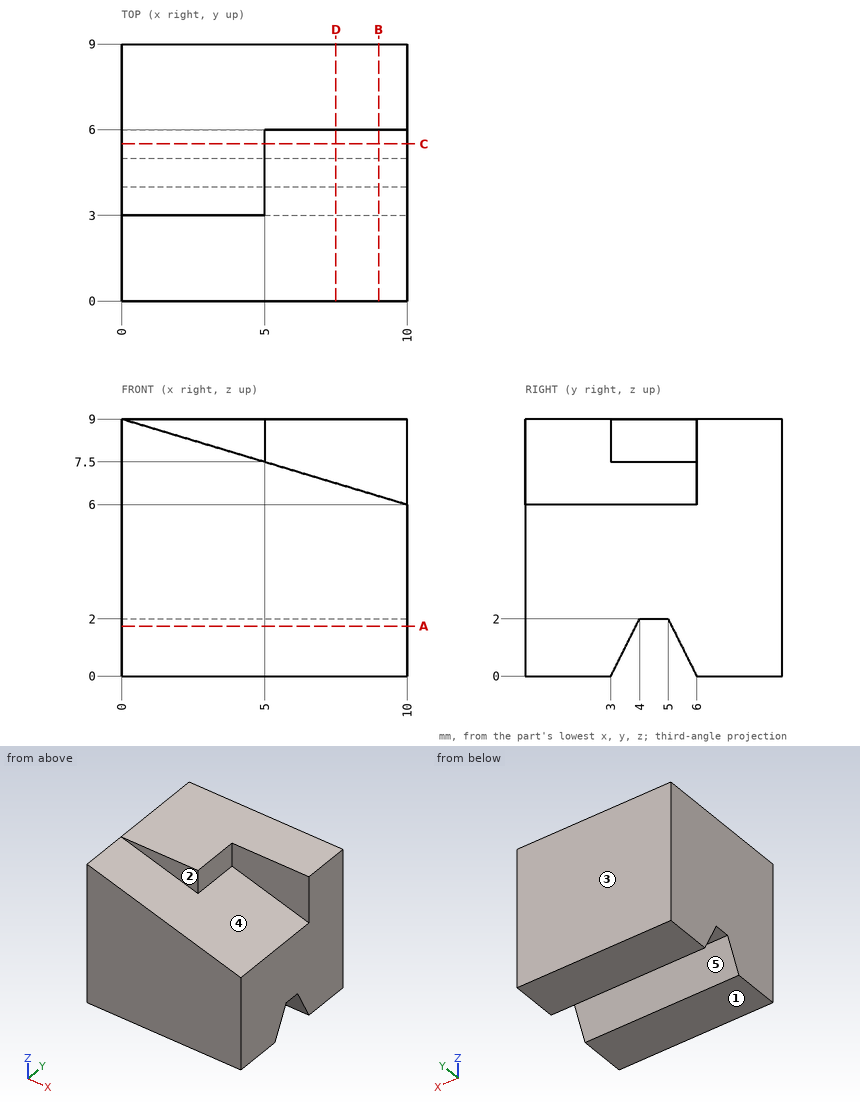
Study the drawing (mm; zero at the part's minimum x, y, z) and answer. A direction names the side the tool comes from. Round coordinates to 2 decimals unless told otherwise and drop trailing zeros. Write each loop counter-clockwise with the first axis right and the second up, starting at its lowest first coordinate (ties: lowest second). Pieces come first, ordered by that corner, then holes. Notation, with made-up numbers: (-22.5, -37.75) -> (29.5, -37.75) arc R10 ccw to (29.5, -26.75) -> close; hole circle Ø2 at (21.5, -35.75). An arc over 180 degrees is marked (long way). Use CSV: the item, a comma, the result in double quotes. Start each with the question number.
(1) The mould has two halves that part along Y. Classify the marked faces 3, 4 and 5: released by +Y, released by -Y, zero draft, split by the parting line, or undercut.
(2) Section B-B on x = 9 is taken. Give the vertices of the cut face in (y, z), then the cut area to 3 significant figures.
(3) Which of the six approach directions +Z, -Z, +X, -X, +Y, -Y give full straight-line access (tool end or side, diameter ignored) to the marked faces 1 and 2?
(4) Section D-D on x = 7.5 is taken. Give the vertices of the cut face in (y, z), then the cut area to 3 significant figures.
(5) Section C-C on y = 5.5 is taken. Give the vertices of the cut face in (x, z).
(6) Section A-A on z = 1.75 is taken. Give the vertices of the cut face in (x, y) (3 decimals).
(7) Consider L1, parallel to Z at x = 0.5, y = 4.5; L2, parallel to Y at x = 2, z = 1; L3, parallel to X at y = 5.75, z = 7.75. Determine where each line is inside the solid, lowest interval first. Write a range as from..to.
(8) Each of these flat-tipped pins is pushed along its axis until it touches: pin 1 (1 mm diameter, centred on y = 5, z = 2, fed in from -X); pin 2 (0.9 mm diameter, centred on x = 7, z = 7.5, fed in from -Y); pin 3 (1.2 mm diameter, centred on y = 5, z = 8.5, fed in from +X); pin 4 (0.5 mm diameter, centred on x = 3.5, y = 4.5, fed in from -Z). Where does it stop, or does it pass through?
A:
1,face 3,"released by +Y"
1,face 4,"zero draft"
1,face 5,"undercut"
2,outline,"(0, 0) -> (3, 0) -> (4, 2) -> (5, 2) -> (6, 0) -> (9, 0) -> (9, 9) -> (6, 9) -> (6, 6.3) -> (0, 6.3) -> close"
2,area,"60.8 mm²"
3,face 1,"-Z, +X, -X, +Y, -Y"
3,face 2,"+Z, +X, -Y"
4,outline,"(0, 0) -> (3, 0) -> (4, 2) -> (5, 2) -> (6, 0) -> (9, 0) -> (9, 9) -> (6, 9) -> (6, 6.75) -> (0, 6.75) -> close"
4,area,"63.5 mm²"
5,outline,"(0, 1) -> (10, 1) -> (10, 6) -> (5, 7.5) -> (5, 9) -> (0, 9) -> close"
6,outline,"(0, 0) -> (10, 0) -> (10, 3.875) -> (0, 3.875) -> close; (0, 5.125) -> (10, 5.125) -> (10, 9) -> (0, 9) -> close"
7,L1,"z = 2..9"
7,L2,"y = 0..3.5, 5.5..9"
7,L3,"x = 0..5"
8,pin 1,"stops at x = 0"
8,pin 2,"stops at y = 6"
8,pin 3,"stops at x = 5"
8,pin 4,"stops at z = 2"
